Can you work these out from the model? Positions are in its coordinate system, mm. Give positions to 0.01 mm unless a question says otherwise; leave off trailing zeros. Write each loop counter-clockwise with the first axis right and the second up, starting at its lowest first coordinate (ties: lowest second). Pieces come first, ordered by that corner, then holes.
from build123d import *

# Parameters (mm, degrees)
BOSS_EXTRUDE1_DEPTH = 2.54


with BuildPart() as part:
    # Sketch1 → Boss-Extrude1 (new body)
    with BuildSketch(Plane(origin=(0, 0, 0), x_dir=(1, 0, 0), z_dir=(0, 1, 0))):
        with BuildLine():
            Line((-5.44692552, -5.352823265), (-2.9654485, 1.134345711))
            Line((-2.9654485, 1.134345711), (-0.48397148, 7.621514688))
            ThreePointArc((-0.48397148, 7.621514688), (-7.132828761, 2.728455313), (-5.44692552, -5.352823265))
        make_face()
        with BuildLine():
            ThreePointArc((-2.9654485, 1.134345711), (1.134345711, 2.9654485), (2.9654485, -1.134345711))
            Line((2.9654485, -1.134345711), (5.44692552, 5.352823265))
            ThreePointArc((5.44692552, 5.352823265), (2.728455313, 7.132828761), (-0.48397148, 7.621514688))
            Line((-0.48397148, 7.621514688), (-2.9654485, 1.134345711))
        make_face()
        with BuildLine():
            Line((0.48397148, -7.621514688), (2.9654485, -1.134345711))
            ThreePointArc((2.9654485, -1.134345711), (-1.134345711, -2.9654485), (-2.9654485, 1.134345711))
            Line((-2.9654485, 1.134345711), (-5.44692552, -5.352823265))
            ThreePointArc((-5.44692552, -5.352823265), (-2.728455313, -7.132828761), (0.48397148, -7.621514688))
        make_face()
        with BuildLine():
            Line((5.44692552, 5.352823265), (2.9654485, -1.134345711))
            Line((2.9654485, -1.134345711), (0.48397148, -7.621514688))
            ThreePointArc((0.48397148, -7.621514688), (4.526523941, -6.150796334), (7.132828761, -2.728455313))
            ThreePointArc((7.132828761, -2.728455313), (7.50979921, -1.387310475), (7.636865491, 0))
            ThreePointArc((7.636865491, 0), (7.068208828, 2.891736243), (5.44692552, 5.352823265))
        make_face()
        with BuildLine():
            ThreePointArc((-0.48397148, 7.621514688), (2.728455313, 7.132828761), (5.44692552, 5.352823265))
            Line((5.44692552, 5.352823265), (6.780173427, 8.83824924))
            Line((6.780173427, 8.83824924), (4.762569184, 8.69478972))
            ThreePointArc((4.762569184, 8.69478972), (1.987351058, 9.970243609), (1.571934345, 12.996139712))
            Line((1.571934345, 12.996139712), (-0.48397148, 7.621514688))
        make_face()
        with BuildLine():
            Line((7.502831345, 10.727448289), (6.780173427, 8.83824924))
            Line((6.780173427, 8.83824924), (24.416674474, 10.092273154))
            Line((24.416674474, 10.092273154), (61.912569184, 12.758377306))
            ThreePointArc((61.912569184, 12.758377306), (64.854387126, 16.150567925), (61.462196506, 19.092385867))
            Line((61.462196506, 19.092385867), (4.312196506, 15.028798281))
            ThreePointArc((4.312196506, 15.028798281), (7.087414633, 13.753344392), (7.502831345, 10.727448289))
        make_face()
        with BuildLine():
            Line((6.780173427, 8.83824924), (5.44692552, 5.352823265))
            ThreePointArc((5.44692552, 5.352823265), (7.068208828, 2.891736243), (7.636865491, 0))
            ThreePointArc((7.636865491, 0), (7.50979921, -1.387310475), (7.132828761, -2.728455313))
            ThreePointArc((7.132828761, -2.728455313), (13.906300834, 6.200799727), (24.416674474, 10.092273154))
            Line((24.416674474, 10.092273154), (6.780173427, 8.83824924))
        make_face()
        with BuildLine():
            Line((4.762569184, 8.69478972), (6.780173427, 8.83824924))
            Line((6.780173427, 8.83824924), (7.502831345, 10.727448289))
            ThreePointArc((7.502831345, 10.727448289), (7.087414633, 13.753344392), (4.312196506, 15.028798281))
            ThreePointArc((4.312196506, 15.028798281), (2.645832454, 14.411825788), (1.571934345, 12.996139712))
            ThreePointArc((1.571934345, 12.996139712), (1.987351058, 9.970243609), (4.762569184, 8.69478972))
        make_face()
        with BuildLine():
            Line((-3.840625768, -18.927036712), (0.48397148, -7.621514688))
            ThreePointArc((0.48397148, -7.621514688), (-2.728455313, -7.132828761), (-5.44692552, -5.352823265))
            Line((-5.44692552, -5.352823265), (-9.771522768, -16.65834529))
            ThreePointArc((-9.771522768, -16.65834529), (-7.940419979, -20.758139501), (-3.840625768, -18.927036712))
        make_face()
    extrude(amount=BOSS_EXTRUDE1_DEPTH)


solid = part.part
(1) Imagine slicing it at B-B, the plane y = 1.1. Write out the boundary of the cut face in (x, z) (3 decimals).
Returned:
outline: (-9.772, 16.658) - (-5.447, 5.353) arc R7.637 ccw to (-0.484, -7.622) - (1.572, -12.996) arc R3.175 ccw to (4.312, -15.029) - (61.462, -19.092) arc R3.175 ccw to (61.913, -12.758) - (24.417, -10.092) arc R20.026 cw to (7.133, 2.728) arc R7.637 ccw to (0.484, 7.622) - (-3.841, 18.927) arc R3.175 ccw to start; hole circle Ø6.35 at (0, 0)
(2) If we mould it in two halves opening along X, with no side actions, what happens to faces 1 (the face through (-1.709, 1.252, 13.353)), 2 (the face through (-8.01, 1.25, 20.73)), 3 (the face through (0.46, 1.25, -3.14)), 4 (the face through (-7.58, 1.25, 10.93))? For each: +X half, -X half, draft (parallel to the pull), parting line (faces both ways), or undercut.
Returned:
face 1: +X half
face 2: parting line
face 3: undercut
face 4: -X half
(3) Will this pin go through, and if not, where does the flat tip stop? P1, Ø10, axis at x = 23, z = -3, coming from the +Y side.
Returned:
P1: passes through
(4) Imagine slicing it at D-D, the plane z = -11. Write out the boundary of the cut face in (x, y), plus the area to 3 significant figures.
Returned:
outline: (0.81, 0) - (37.18, 0) - (37.18, 2.54) - (0.81, 2.54) - close
area: 92.4 mm2
(5) If I drill on L1, parallel to X at y = 0.95, z = 0 (3 decimals); L2, parallel to X at y = 2.35, z = 0.5; L3, parallel to Z at x = 12.5, y = 0.25, over which ranges is the centre line in solid material (lowest first)?
Returned:
L1: x = -7.637 to -3.175, 3.175 to 8.42
L2: x = -7.62 to -3.14, 3.14 to 8.15
L3: z = -15.61 to -5.06
(6) Imagine slicing it at C-C, the plane x = 46. Write out the boundary of the cut face in (y, z).
Returned:
outline: (0, -17.99) - (2.54, -17.99) - (2.54, -11.63) - (0, -11.63) - close
(7) Imagine slicing it at A-A, the plane z = -2. Write out the boundary of the cut face in (x, y), plus the area to 3 significant figures.
Returned:
outline: (-7.37, 0) - (-2.47, 0) - (-2.47, 2.54) - (-7.37, 2.54) - close; (2.47, 0) - (9.72, 0) - (9.72, 2.54) - (2.47, 2.54) - close
area: 30.9 mm2
